CAD build for the part. Positions are in the model's coordinates, mm. Round coordinates to 2 decimals unless told otherwise and drop trailing zeros. Write each loop counter-clockwise with the first axis right and the second up, starting at its lowest first coordinate (ties: lowest second). Pieces come first, ordered by that corner, then holes. Notation, with made-up numbers: (-9, -11.75) - (35, -11.75) arc R16 ccw to (35, 1.25) - close; hole circle Ø4 at (52.5, -29). An arc over 180 degrees is marked (long way). Answer in a Markdown table with one row per item.
```python
from build123d import *

# Parameters (mm, degrees)
SKETCH1_R           = 1.6
BOSS_EXTRUDE1_DEPTH = 5


with BuildPart() as part:
    # Sketch1 → Boss-Extrude1 (new body)
    with BuildSketch(Plane(origin=(0, 0, 0), x_dir=(1, 0, 0), z_dir=(0, 1, 0))):
        with BuildLine():
            Line((-66, -60), (66, -60))
            ThreePointArc((66, -60), (68.828427125, -58.828427125), (70, -56))
            Line((70, -56), (70, 56))
            ThreePointArc((70, 56), (68.828427125, 58.828427125), (66, 60))
            Line((66, 60), (-66, 60))
            ThreePointArc((-66, 60), (-68.828427125, 58.828427125), (-70, 56))
            Line((-70, 56), (-70, -56))
            ThreePointArc((-70, -56), (-68.828427125, -58.828427125), (-66, -60))
        make_face()
        with Locations((-66, 56)):
            Circle(SKETCH1_R, mode=Mode.SUBTRACT)
        with Locations((-66, -56)):
            Circle(SKETCH1_R, mode=Mode.SUBTRACT)
        with Locations((66, -56)):
            Circle(SKETCH1_R, mode=Mode.SUBTRACT)
        with Locations((66, 56)):
            Circle(SKETCH1_R, mode=Mode.SUBTRACT)
        with Locations((-66, -20)):
            Circle(SKETCH1_R, mode=Mode.SUBTRACT)
        with Locations((66, -20)):
            Circle(SKETCH1_R, mode=Mode.SUBTRACT)
        with Locations((-66, 20)):
            Circle(SKETCH1_R, mode=Mode.SUBTRACT)
        with Locations((66, 20)):
            Circle(SKETCH1_R, mode=Mode.SUBTRACT)
        with Locations((-21, -56)):
            Circle(SKETCH1_R, mode=Mode.SUBTRACT)
        with Locations((21, -56)):
            Circle(SKETCH1_R, mode=Mode.SUBTRACT)
        with Locations((-26.5, 56)):
            Circle(SKETCH1_R, mode=Mode.SUBTRACT)
        with Locations((26.5, 56)):
            Circle(SKETCH1_R, mode=Mode.SUBTRACT)
    extrude(amount=BOSS_EXTRUDE1_DEPTH)


solid = part.part
```
Q1. Flat gauge pin, fed straight in: pin 1 (1.9 mm diameter, centred on x = -21, z = 56, fed in from -Y). Where does the tip first touch, or does it go through?
Computed:
| item | result |
|---|---|
| pin 1 | passes through |
Q2. Drill centre lines: line 1 (X direction, y = 1.3, z = -56); line 2 (Z direction, x = 66, y = 3.15); line 3 (X direction, y = 3.5, z = 56). Where is each one in solid material? Low to high.
Computed:
| item | result |
|---|---|
| line 1 | x = -70 to -67.6, -64.4 to -28.1, -24.9 to 24.9, 28.1 to 64.4, 67.6 to 70 |
| line 2 | z = -60 to -57.6, -54.4 to -21.6, -18.4 to 18.4, 21.6 to 54.4, 57.6 to 60 |
| line 3 | x = -70 to -67.6, -64.4 to -22.6, -19.4 to 19.4, 22.6 to 64.4, 67.6 to 70 |
Q3. Saw through at A-A on z = -20. List the corners of the cut face in (x, y), then the cut area to 3 significant figures.
Computed:
| item | result |
|---|---|
| outline | (-70, 0) - (-67.6, 0) - (-67.6, 5) - (-70, 5) - close; (-64.4, 0) - (64.4, 0) - (64.4, 5) - (-64.4, 5) - close; (67.6, 0) - (70, 0) - (70, 5) - (67.6, 5) - close |
| area | 668 mm2 |
Q4. Pull direction Z, two halves, no side cores. Call faces 1 (the cylindrical face through (67.526, 2.465, 55.519)), 2 (the flat face through (-1, 2, 60)), 3 (the flat face through (70, 2, 1)): released by +Z, released by -Z, zero draft, split by the parting line, or undercut.
Computed:
| item | result |
|---|---|
| face 1 | undercut |
| face 2 | released by +Z |
| face 3 | zero draft |
Q5. Saw through at B-B on x = -21. List the corners of the cut face in (y, z), then the cut area to 3 significant figures.
Computed:
| item | result |
|---|---|
| outline | (0, -60) - (5, -60) - (5, 54.4) - (0, 54.4) - close; (0, 57.6) - (5, 57.6) - (5, 60) - (0, 60) - close |
| area | 584 mm2 |
